from build123d import *

# Parameters (mm, degrees)
SKETCH1_W           = 43.5
SKETCH1_H           = 43.5
SKETCH1_R           = 1.5
BOSS_EXTRUDE1_DEPTH = 1.5
SKETCH2_R           = 2.5
SKETCH2_R_2         = 1.5
CUT_EXTRUDE1_DEPTH  = 0.0001
SKETCH3_R           = 2.5
SKETCH3_R_2         = 1.5
CUT_EXTRUDE2_DEPTH  = 0.002
SKETCH4_W           = 7
SKETCH4_H           = 0.5
CUT_EXTRUDE4_DEPTH  = 0.0001
SKETCH6_W           = 8
SKETCH6_H           = 15
SKETCH6_W_2         = 10
SKETCH6_H_2         = 8
CUT_EXTRUDE5_DEPTH  = 0.0001
SKETCH8_R           = 4
CUT_EXTRUDE6_DEPTH  = 0.0001
SKETCH9_W           = 14.5
SKETCH9_H           = 4
CUT_EXTRUDE7_DEPTH  = 0.0001
SKETCH10_W          = 5
SKETCH10_H          = 15.24
CUT_EXTRUDE8_DEPTH  = 0.0001
SKETCH11_R          = 4
SKETCH11_W          = 14.5
SKETCH11_H          = 4
CUT_EXTRUDE9_DEPTH  = 0.0001
CUT_EXTRUDE10_DEPTH = 0.0001
SKETCH13_W          = 6.9
SKETCH13_H          = 10
CUT_EXTRUDE11_DEPTH = 0.0001


with BuildPart() as part:
    # Sketch1 → Boss-Extrude1 (new body)
    with BuildSketch(Plane.XY):
        Rectangle(SKETCH1_W, SKETCH1_H)
        with Locations((-18.758938316, 18.758938316)):
            Circle(SKETCH1_R, mode=Mode.SUBTRACT)
        with Locations((18.758938316, 18.758938316)):
            Circle(SKETCH1_R, mode=Mode.SUBTRACT)
        with Locations((18.758938316, -18.758938316)):
            Circle(SKETCH1_R, mode=Mode.SUBTRACT)
        with Locations((-18.758938316, -18.758938316)):
            Circle(SKETCH1_R, mode=Mode.SUBTRACT)
    extrude(amount=BOSS_EXTRUDE1_DEPTH)

    # Sketch2 → Cut-Extrude1 (cut)
    with BuildSketch(Plane.XY.offset(1.5)):
        with Locations((-18.758938316, 18.758938316)):
            Circle(SKETCH2_R)
        with Locations((-18.758938316, 18.758938316)):
            Circle(SKETCH2_R_2, mode=Mode.SUBTRACT)
        with Locations((18.758938316, 18.758938316)):
            Circle(SKETCH2_R)
        with Locations((18.758938316, 18.758938316)):
            Circle(SKETCH2_R_2, mode=Mode.SUBTRACT)
        with Locations((18.758938316, -18.758938316)):
            Circle(SKETCH2_R)
        with Locations((18.758938316, -18.758938316)):
            Circle(SKETCH2_R_2, mode=Mode.SUBTRACT)
        with Locations((-18.758938316, -18.758938316)):
            Circle(SKETCH2_R)
        with Locations((-18.758938316, -18.758938316)):
            Circle(SKETCH2_R_2, mode=Mode.SUBTRACT)
    extrude(amount=-CUT_EXTRUDE1_DEPTH, mode=Mode.SUBTRACT)

    # Sketch3 → Cut-Extrude2 (cut)
    with BuildSketch(Plane(origin=(0, 0, 0), x_dir=(-1, 0, 0), z_dir=(0, 0, -1))):
        with Locations((-18.758938316, -18.758938316)):
            Circle(SKETCH3_R)
        with Locations((-18.758938316, -18.758938316)):
            Circle(SKETCH3_R_2, mode=Mode.SUBTRACT)
        with Locations((-18.758938316, 18.758938316)):
            Circle(SKETCH3_R)
        with Locations((-18.758938316, 18.758938316)):
            Circle(SKETCH3_R_2, mode=Mode.SUBTRACT)
        with Locations((18.758938316, 18.758938316)):
            Circle(SKETCH3_R)
        with Locations((18.758938316, 18.758938316)):
            Circle(SKETCH3_R_2, mode=Mode.SUBTRACT)
        with Locations((18.758938316, -18.758938316)):
            Circle(SKETCH3_R)
        with Locations((18.758938316, -18.758938316)):
            Circle(SKETCH3_R_2, mode=Mode.SUBTRACT)
    extrude(amount=-CUT_EXTRUDE2_DEPTH, mode=Mode.SUBTRACT)

    # Sketch4 → Cut-Extrude4 (cut)
    with BuildSketch(Plane.XY.offset(1.5)):
        Polygon((14.95, 11), (21.65, 11), (21.65, 11.5), (12.65, 11.5), (12.65, 11), (12.65, -11), (12.65, -11.5), (21.65, -11.5), (21.65, -11), (14.95, -11), (14.95, -7), (21.65, -7), (21.65, -6.5), (13.55, -6.5), (13.55, -2.5), (21.65, -2.5), (21.65, -2), (14.95, -2), (14.95, 2), (21.65, 2), (21.65, 2.5), (13.55, 2.5), (13.55, 6.5), (21.65, 6.5), (21.65, 7), (14.95, 7), align=None)
        with Locations((9.15, 11.25)):
            Rectangle(SKETCH4_W, SKETCH4_H)
        with Locations((9.15, -11.25)):
            Rectangle(SKETCH4_W, SKETCH4_H)
    extrude(amount=-CUT_EXTRUDE4_DEPTH, mode=Mode.SUBTRACT)

    # Sketch6 → Cut-Extrude5 (cut)
    with BuildSketch(Plane.XY.offset(1.5)):
        with Locations((-17.15, 7.65)):
            Rectangle(SKETCH6_W, SKETCH6_H)
        with Locations((-7.55, 17.15)):
            Rectangle(SKETCH6_W_2, SKETCH6_H_2)
        with Locations((-7.55, -17.15)):
            Rectangle(SKETCH6_W_2, SKETCH6_H_2)
    extrude(amount=-CUT_EXTRUDE5_DEPTH, mode=Mode.SUBTRACT)

    # Sketch8 → Cut-Extrude6 (cut)
    with BuildSketch(Plane.XY.offset(1.5)):
        Polygon((-0.05, 7.98), (-2.52, 10.45), (-5.88, 10.45), (-8.35, 7.98), (-8.35, 2.15), (-0.05, 2.15), align=None)
        with Locations((-4.2, 6.3)):
            Circle(SKETCH8_R, mode=Mode.SUBTRACT)
    extrude(amount=-CUT_EXTRUDE6_DEPTH, mode=Mode.SUBTRACT)

    # Sketch9 → Cut-Extrude7 (cut)
    with BuildSketch(Plane.XY.offset(1.5)):
        with Locations((7.5, 18.05)):
            Rectangle(SKETCH9_W, SKETCH9_H)
    extrude(amount=-CUT_EXTRUDE7_DEPTH, mode=Mode.SUBTRACT)

    # Sketch10 → Cut-Extrude8 (cut)
    with BuildSketch(Plane.XY.offset(1.5)):
        with Locations((-17.85, -8.33)):
            Rectangle(SKETCH10_W, SKETCH10_H)
    extrude(amount=-CUT_EXTRUDE8_DEPTH, mode=Mode.SUBTRACT)

    # Sketch11 → Cut-Extrude9 (cut)
    with BuildSketch(Plane.XY.offset(1.5)):
        Polygon((-9.42, -2.55), (-12.78, -2.55), (-15.25, -5.02), (-15.25, -10.85), (-6.95, -10.85), (-6.95, -5.02), align=None)
        with Locations((-11.1, -6.7)):
            Circle(SKETCH11_R, mode=Mode.SUBTRACT)
        with Locations((7.5, -18.05)):
            Rectangle(SKETCH11_W, SKETCH11_H)
    extrude(amount=-CUT_EXTRUDE9_DEPTH, mode=Mode.SUBTRACT)

    # Sketch12 → Cut-Extrude10 (cut)
    with BuildSketch(Plane.XY.offset(1.5)):
        Polygon((-9.81, 11.04), (-10.52, 11.75), (-11.64, 11.75), (-12.35, 11.04), (-12.35, 7.46), (-11.64, 6.75), (-10.52, 6.75), (-9.81, 7.46), align=None)
    extrude(amount=-CUT_EXTRUDE10_DEPTH, mode=Mode.SUBTRACT)

    # Sketch13 → Cut-Extrude11 (cut)
    with BuildSketch(Plane.XY.offset(1.5)):
        with Locations((-2.5, -5.75)):
            Rectangle(SKETCH13_W, SKETCH13_H)
    extrude(amount=-CUT_EXTRUDE11_DEPTH, mode=Mode.SUBTRACT)


solid = part.part
Could you check a few things on this model? Use its own coordinates, in mm. Give positions to 0.01 mm unless a question says otherwise; leave off trailing zeros. Return JSON: item names as keys, results as strings.
Item 1: I need wall thicknesses on L1, parallel to X at y = -18, z = 1.05; L2, parallel to X at y = 17.5, z = 0.9. Which ranges of each line are inside material? Lowest first, please. Write a range as from..to.
Geometry results:
{"L1": "x = -21.75..-20.05, -17.47..17.47, 20.05..21.75", "L2": "x = -21.75..-19.57, -17.94..17.94, 19.57..21.75"}
Item 2: I'm going to push a flat-ended pin straight in: pin 1 (4 mm diameter, centred on x = -18.76, y = 18.76, fed in from -Z). Where does the tip first touch, or does it pass through?
Geometry results:
{"pin 1": "stops at z = 0"}
Item 3: If we section it at A-A on x = 19.5: Count the separate pieces of the cut face and the enclosed holes in it, plus the area to 3 significant figures.
Geometry results:
{"separate pieces": "3", "enclosed holes": "0", "area": "57.4 mm²"}
Item 4: We'd pull the mould along X, two halves only. Please class faces 1 (the cylindrical face through (18.434, 17.295, 0.74)), 2 (the flat face through (-17, -19, 1.5)): +X half, -X half, draft (parallel to the pull), parting line (faces both ways), or undercut.
Geometry results:
{"face 1": "undercut", "face 2": "draft"}
